Part model, mm, in its own coordinate system. A direction names the side the tool comes from. Coordinates: 2 decimals unless noted, no trailing zeros. Loops run counter-clockwise (first coordinate to the right, second up) from the corner with the lowest first, then second, coordinate; pieces in that order, holes last. Notation, with made-up numbers: (31, 13.5) - (58, 13.5) arc R31 cw to (58, 50.5) - close; hole circle Ø2 at (52.25, 68). An arc over 180 degrees is marked (long way). Use a Markdown table: item, result. Add a question column.
1. Wall check: probe 1 along Y at (x, z) = (-37, -0.25); probe 2 along Y at (x, z) = (-38, -14); probe 3 along X at (y, z) = (-35.5, -8). Give the ranges that are in metal, low to high. Write a range as [from, to].
2. Band-saw the part on C-C, the plane y = 0. Give the cut face in (x, z), plus the area to 3 significant figures.
3. 3-axis set-ups, long thin cutter, end or side, ignore diameter. For faces 1 (the flat face through (7, 1, -15.24)), 2 (the cylindrical face through (-5.291, -40.294, 1.252)): which of +Z, -Z, +X, -X, +Y, -Y reach the whole face in a straight line?
4. Drop a flat-ended pin along its axis: pin 1 (23 mm diameter, centred on x = 41.31, y = 41.31, fed in from +Z). Give the stop position or say it passes through.
5. Pull direction Y, two halves, no side cores. Call faces 3 (the cylindrical face through (40.152, -32.495, -7.513)), 4 (the cylindrical face through (-52.983, -54.095, -6.261)), 5 (the flat face through (-55.88, -1, -6)): pulls with the +Y half, pulls with the -Y half, needs draft (parallel to the pull), parting line crosses it, or undercut.
6. Band-saw the part on D-D, the plane x = 56. Give the cut face in (y, z), plus the area to 3 significant figures.
7. Band-saw the part on A-A, the plane x = 0. Give the cut face in (y, z), plus the area to 3 significant figures.
8. Band-saw the part on B-B, the plane z = -2.75. Give the cut face in (x, y), plus the area to 3 significant figures.
Autodesk Inventor part; units mm, degrees
ref_plane "YZ Plane" through (0, 0, 0) normal (1, 0, 0) x (0, 1, 0)
ref_plane "XZ Plane" through (0, 0, 0) normal (0, 1, 0) x (-1, 0, 0)
ref_plane "XY Plane" through (0, 0, 0) normal (0, 0, 1) x (1, 0, 0)
sketch "Sketch1" plane through (0, 0, 0) normal (0, 0, 1) x (1, 0, 0)
  line L0 (-45.72, 57.15) -> (60.96, 57.15)
  line L1 (71.12, 46.99) -> (71.12, -46.99)
  line L2 (60.96, -57.15) -> (-45.72, -57.15)
  line L3 (-55.88, -46.99) -> (-55.88, 46.99)
  line L4 (-85.7425, 0) -> (99.7187, 0)
  line L5 (0, -82.9559) -> (0, 82.9559)
  circle A0 centre (0, 0) radius 40.64
  circle A1 centre (0, 0) radius 58.42 construction
  line L6 (0, 0) -> (-59.2481, 59.2481) construction
  circle A2 centre (-41.3092, 41.3092) radius 8.89
  circle A3 centre (-41.3092, -41.3092) radius 8.89
  circle A4 centre (41.3092, -41.3092) radius 8.89
  circle A5 centre (41.3092, 41.3092) radius 8.89
  arc A6 (-45.72, 57.15) -> (-55.88, 46.99) centre (-45.72, 46.99) ccw
  arc A7 (71.12, 46.99) -> (60.96, 57.15) centre (60.96, 46.99) ccw
  arc A8 (60.96, -57.15) -> (71.12, -46.99) centre (60.96, -46.99) ccw
  arc A9 (-55.88, -46.99) -> (-45.72, -57.15) centre (-45.72, -46.99) ccw
  point P0 (71.12, -57.15)
  point P1 (71.12, 57.15)
  point P2 (-55.88, -57.15)
  point P3 (71.12, 0)
  dimension "d4" = 116.84
  dimension "d0" = 127
  dimension "d1" = 114.3
  dimension "d2" = 55.88
  dimension "d3" = 81.28
  dimension "d5" = 45
  dimension "d6" = 17.78
  dimension "d9" = 360
  dimension "d11" = 10.16
  dimension "d12" = 59.2481
extrude "Extrusion1" add sketch "Sketch1" against normal blind 15.24
extrude "Extrusion2" add sketch "Sketch1" along normal blind 5.08 contours A0 L4 L5 | L5 L4 A0 | L5 A0 L4 | L4 A0 L5
chamfer "Chamfer1" distance 2.54 angle 45 1 edges at (-40.64, 0, 5.08) measured on face at (4.2922, -0.5549, 5.08)
fillet "Fillet1" radius 2.54 8 edges at (68.1442, 54.1742, -15.24) (71.12, 0, -15.24) (68.1442, -54.1742, -15.24) (7.62, -57.15, -15.24) (-52.9042, -54.1742, -15.24) (-55.88, 0, -15.24) (-52.9042, 54.1742, -15.24) (7.62, 57.15, -15.24)
equation "\"BendRadius\" = Thickness"
equation "\"BendReliefWidth\" = Thickness"
equation "\"BendReliefDepth\" = 0.5 * Thickness"
equation "\"CornerReliefSize\" = 4 * Thickness"
equation "\"MinimumRemnant\" = 2 * Thickness"
equation "\"TransitionRadius\" = BendRadius"
equation "\"JacobiRadiusSize\" = BendRadius"
equation "\"GapSize\" = Thickness"
properties part number "cylinder head" material "Aluminum 6061"
Geometry check:
| question | item | result |
|---|---|---|
| 1 | probe 1 | y = [-57.15, -49.08], [-33.53, 33.53], [49.08, 57.15] |
| 1 | probe 2 | y = [-56.79, -49.56], [-33.06, 33.06], [49.56, 56.79] |
| 1 | probe 3 | x = [-55.88, -48.04], [-34.58, 34.58], [48.04, 71.12] |
| 2 | outline | (-55.88, -12.7) arc R2.54 ccw to (-53.34, -15.24) - (68.58, -15.24) arc R2.54 ccw to (71.12, -12.7) - (71.12, 0) - (40.64, 0) - (40.64, 2.54) - (38.1, 5.08) - (-38.1, 5.08) - (-40.64, 2.54) - (-40.64, 0) - (-55.88, 0) - close |
| 2 | area | 2,340 mm^2 |
| 3 | face 1 | -Z, +X, -X, +Y, -Y |
| 3 | face 2 | +Z |
| 4 | pin 1 | stops at z = 0 |
| 5 | face 3 | undercut |
| 5 | face 4 | pulls with the -Y half |
| 5 | face 5 | needs draft |
| 6 | outline | (-57.15, -12.7) arc R2.54 ccw to (-54.61, -15.24) - (54.61, -15.24) arc R2.54 ccw to (57.15, -12.7) - (57.15, 0) - (-57.15, 0) - close |
| 6 | area | 1,740 mm^2 |
| 7 | outline | (-57.15, -12.7) arc R2.54 ccw to (-54.61, -15.24) - (54.61, -15.24) arc R2.54 ccw to (57.15, -12.7) - (57.15, 0) - (40.64, 0) - (40.64, 2.54) - (38.1, 5.08) - (-38.1, 5.08) - (-40.64, 2.54) - (-40.64, 0) - (-57.15, 0) - close |
| 7 | area | 2,150 mm^2 |
| 8 | outline | (-55.88, -46.99) arc R10.16 ccw to (-45.72, -57.15) - (60.96, -57.15) arc R10.16 ccw to (71.12, -46.99) - (71.12, 46.99) arc R10.16 ccw to (60.96, 57.15) - (-45.72, 57.15) arc R10.16 ccw to (-55.88, 46.99) - close; hole circle Ø17.78 at (-41.31, -41.31); hole circle Ø17.78 at (-41.31, 41.31); hole circle Ø17.78 at (41.31, -41.31); hole circle Ø17.78 at (41.31, 41.31) |
| 8 | area | 13,400 mm^2 |
